```python
from build123d import *

# Parameters (mm, degrees)
PAD002_DEPTH    = 7
PAD003_DEPTH    = 7
PAD004_DEPTH    = 7
SKETCH011_R     = 5.25
PAD005_DEPTH    = 3
SKETCH012_R     = 5.125
POCKET002_DEPTH = 25.001


with BuildPart() as part:
    # Sketch008 (on DatumPlane) → Pad002 (new body)
    with BuildSketch(Plane(origin=(0, 0, 0), x_dir=(-0.8660254038, -0.5, 0), z_dir=(-0.5, 0.8660254038, 0))):
        Polygon((-3, 0), (3, 0), (3, -15), (2, -15), (2, -20), (1, -20), (1, -25), (-1, -25), (-1, -20), (-2, -20), (-2, -15), (-3, -15), align=None)
    extrude(amount=PAD002_DEPTH)

    # Sketch009 (on DatumPlane) → Pad003 (join)
    with BuildSketch(Plane(origin=(0, 0, 0), x_dir=(0.8660254038, -0.5, 0), z_dir=(-0.5, -0.8660254038, 0))):
        Polygon((-3, 0), (3, 0), (3, -15), (2, -15), (2, -20), (1, -20), (1, -25), (-1, -25), (-1, -20), (-2, -20), (-2, -15), (-3, -15), align=None)
    extrude(amount=PAD003_DEPTH)

    # Sketch010 → Pad004 (join)
    with BuildSketch(Plane.YZ):
        Polygon((-3, 0), (3, 0), (3, -15), (2, -15), (2, -20), (1, -20), (1, -25), (-1, -25), (-1, -20), (-2, -20), (-2, -15), (-3, -15), align=None)
    extrude(amount=PAD004_DEPTH)

    # Sketch011 → Pad005 (join)
    with BuildSketch(Plane.XY):
        Circle(SKETCH011_R)
    extrude(amount=-PAD005_DEPTH)

    # Sketch012 → Pocket002 (cut, through all)
    with BuildSketch(Plane.XY):
        Circle(SKETCH012_R)
    extrude(amount=-POCKET002_DEPTH, mode=Mode.SUBTRACT)


solid = part.part
```
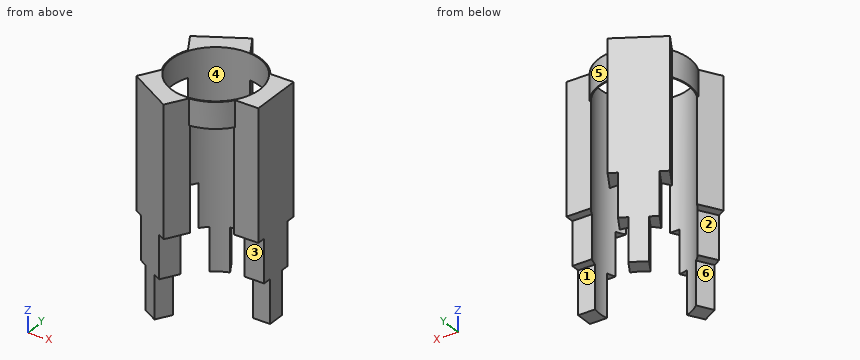
For this review, take the finished solid that the model builds, in its own axes (mm). Face numbers are marked on the shaded views. A direction names the side the tool comes from. Coordinates: 2 decimals unless noted, no trailing zeros. Order: outer loops, then holes, each group sorted by start corner. A loop starts at its lowest first (then second) coordinate and runs counter-clockwise, first axis right, second up. Notation, with made-up numbers: (36.25, 16.25) -> (94.25, 16.25) arc R32 ccw to (94.25, 42.25) -> close; hole circle Ø2 at (68, 78.25). An arc over 180 degrees is marked (long way). Answer as CSV lines item,"result".
Q1. For the marked faces 1, 2 and 3, list the 3-axis set-ups (+Z, -Z, +X, -X, +Y, -Y) from which the entire face can be reached by the end or side of a thin tool; tool diameter is ignored.
Model answer:
face 1,"-Z, +X, -X, +Y"
face 2,"-Z, -X"
face 3,"-Z, +X, -X, -Y"
Q2. Wall thickness on line 1 along X through (y, z) = (1, -8.25); line 2 along X through (y, z) = (0, -6) (3 decimals); line 3 along X through (y, z) = (-4, -1.5): over which ranges is each line inside the solid? List them lowest first. Write a range as [from, to].
Model answer:
line 1,"x = [5.03, 7]"
line 2,"x = [5.125, 7]"
line 3,"x = [-5.77, -3.2], [3.2, 3.4]"
Q3. We need section B-B (y = 0). State the section outline as (x, z) points (3 decimals), plus the area to 4 significant figures.
Model answer:
outline,"(-5.25, -3) -> (-5.125, -3) -> (-5.125, 0) -> (-5.25, 0) -> close; (5.125, -25) -> (7, -25) -> (7, 0) -> (5.125, 0) -> close"
area,"47.25 mm2"
Q4. Draft analysis for pull direction X (two halves, no side actions). For the marked faces 4, 5 and 6, state which applies: released by +X, released by -X, zero draft, split by the parting line, or undercut.
Model answer:
face 4,"undercut"
face 5,"released by +X"
face 6,"released by -X"
Q5. We need section C-C (x = 0). State the section outline as (y, z) points (3 decimals), plus the area to 4 significant figures.
Model answer:
outline,"(-6, -15) -> (-5.125, -15) -> (-5.125, 0) -> (-6, 0) -> close; (5.125, -15) -> (6, -15) -> (6, 0) -> (5.125, 0) -> close"
area,"26.25 mm2"
Q6. Clearance check with flat-ended pins moving along their axes: pin 1 Ø6 at (x, z) = (3, -20.5) entering from +Y; pin 2 Ø6 at (y, z) = (-5, -22) entering from -X; pin 3 Ø0.9 at (x, z) = (5.5, -6) entering from +Y. State where each tip first meets the part, or that it passes through.
Model answer:
pin 1,"stops at y = 2"
pin 2,"stops at x = -5.23"
pin 3,"stops at y = 3"
Q7. We need section A-A (z = -21). Count the separate pieces of the cut face and the enclosed holes in it, plus the area to 3 significant figures.
Model answer:
separate pieces,"3"
enclosed holes,"0"
area,"11.4 mm2"
Q8. We need section D-D (z = -1.75). State the section outline as (x, y) points (3 decimals), plus the area to 3 significant figures.
Model answer:
outline,"(-6.098, -4.562) -> (-0.902, -7.562) -> (0.444, -5.231) arc R5.25 ccw to (4.308, -3) -> (7, -3) -> (7, 3) -> (4.308, 3) arc R5.25 ccw to (0.444, 5.231) -> (-0.902, 7.562) -> (-6.098, 4.562) -> (-4.752, 2.231) arc R5.25 ccw to (-4.752, -2.231) -> close; hole circle Ø10.25 at (0, 0)"
area,"41.0 mm2"
